Verification items for this drawing (mm, ordinates from the low corner). A direction names the side the tool comes from. Round coordinates to 2 decimals unless told otherwise and drop trailing zeros. Write each loop counter-clockwise with the first axis right and the second up, starting at its lowest first coordinate (ties: lowest second). Pieces come first, ordered by that corner, then holes. Notation, with made-up numbers: (77.25, -23.5) -> (123.25, -23.5) arc R21 cw to (123.25, -7.5) -> close; hole circle Ø8 at (83.5, -37). An arc over 180 degrees is marked (long way). One line per question, with ' | ' between items.
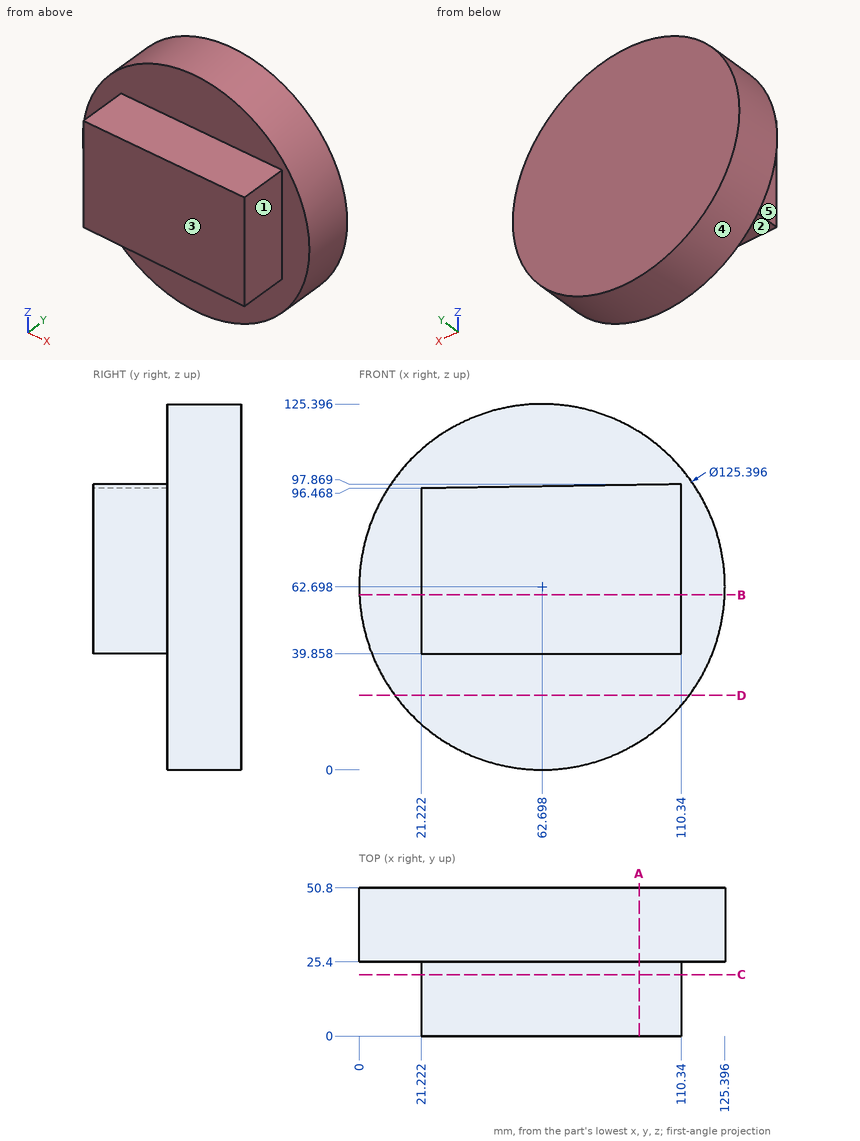
(1) Access from +Z, -Z, +X, -X, +Y, -Y to the whole of each face (thin tool, end or side, straight path). Record for the marked faces 1, 2, 3, 4 and 5.
Resolved:
face 1: +Z, -Z, +X, -Y | face 2: -Z, +X, -X, -Y | face 3: +Z, -Z, +X, -X, -Y | face 4: +Y, -Y | face 5: +Z, -Z, -X, -Y
(2) Sectioned sample at D-D on z = 25.5. Record the cut outline in (x, y), then the cut area to 3 significant figures.
Resolved:
outline: (12.23, 25.4) -> (113.17, 25.4) -> (113.17, 50.8) -> (12.23, 50.8) -> close | area: 2,560 mm2
(3) Sectioned sample at C-C on y = 21. Record the cut outline in (x, z), then the cut area to 3 significant figures.
Resolved:
outline: (21.22, 39.86) -> (110.34, 39.86) -> (110.34, 97.87) -> (21.22, 96.47) -> close | area: 5,110 mm2
(4) Sectioned sample at A-A on x = 96. Record the cut outline in (y, z) (1 decimal).
Resolved:
outline: (0, 39.9) -> (25.4, 39.9) -> (25.4, 9.6) -> (50.8, 9.6) -> (50.8, 115.8) -> (25.4, 115.8) -> (25.4, 97.6) -> (0, 97.6) -> close
(5) Material ranges on line 1 (X direction, y = 7.5, z = 60.5); line 2 (Y direction, x = 68, z = 11); line 3 (Z direction, x = 63.5, y = 34) (1 decimal), recorded low to high.
Resolved:
line 1: x = 21.22 to 110.34 | line 2: y = 25.4 to 50.8 | line 3: z = 0 to 125.4
(6) Go/stop test with flat-tipped pins: pin 1 (1.5 mm diameter, centred on y = 33.5, z = 39.5, fed in from -X); pin 2 (1.5 mm diameter, centred on x = 48.5, y = 13, fed in from +Z); pin 3 (20.5 mm diameter, centred on y = 13, z = 55, fed in from -X). Record where each tip stops, or that it passes through.
Resolved:
pin 1: stops at x = 4.16 | pin 2: stops at z = 96.91 | pin 3: stops at x = 21.22
(7) Sectioned sample at B-B on z = 60. Record the cut outline in (x, y).
Resolved:
outline: (0.06, 25.4) -> (21.22, 25.4) -> (21.22, 0) -> (110.34, 0) -> (110.34, 25.4) -> (125.34, 25.4) -> (125.34, 50.8) -> (0.06, 50.8) -> close
